from build123d import *

# Parameters (mm, degrees)
SKETCH_1_R               = 72.5
SKETCH_1_R_2             = 65
EXTRUDE_1_DEPTH          = 1
SKETCH_2_W               = 1
SKETCH_2_H               = 0.5
SKETCH_3_R               = 67.173254354
CUT_EXTRUDE_1_DEPTH      = 500
EXTRUDE_START            = 6
SKETCH_4_R               = 69.173254354
SKETCH_4_R_2             = 67.173254354
EXTRUDE_2_DEPTH          = 6
SKETCH_9_R               = 3
CUT_EXTRUDE_3_DEPTH      = 50
PATTERN_CIRCULAR_1_COUNT = 8
EXTRUDE_4_REACH          = 105.351
SKETCH_10_R              = 64.083899557
SKETCH_10_R_2            = 42.5
SKETCH_11_R              = 3
CUT_EXTRUDE_4_DEPTH      = 50
PATTERN_CIRCULAR_2_COUNT = 8
EXTRUDE_START_2          = -1
SKETCH_13_R              = 3
SKETCH_13_R_2            = 1.5
EXTRUDE_5_DEPTH          = 1
PATTERN_CIRCULAR_3_COUNT = 8
CUT_EXTRUDE_5_DEPTH      = 1
PATTERN_CIRCULAR_4_COUNT = 4


with BuildPart() as part:
    # 草图1 → 凸台-拉伸1 (new body)
    with BuildSketch(Plane(origin=(0, 0, 0), x_dir=(1, 0, 0), z_dir=(0, 1, 0))):
        with Locations(Location((0, 0, 0), (0, 0, 270))):
            Circle(SKETCH_1_R)
        with Locations(Location((0, 0, 0), (0, 0, 270))):
            Circle(SKETCH_1_R_2, mode=Mode.SUBTRACT)
    extrude(amount=EXTRUDE_1_DEPTH)

    # 草图2 → 旋转1 (revolve)
    with BuildSketch(Plane.XY, mode=Mode.PRIVATE) as revolve_1_sk:
        with Locations((-72, 1.25)):
            Rectangle(SKETCH_2_W, SKETCH_2_H)
    revolve(revolve_1_sk.sketch.rotate(Axis((0, 15.807831018, 0), (0, -1, 0)), 270), axis=Axis((0, 15.807831018, 0), (0, -1, 0)))

    # 草图3 → 切除-拉伸1 (cut)
    with BuildSketch(Plane(origin=(0, 1, 0), x_dir=(1, 0, 0), z_dir=(0, 1, 0))):
        with Locations(Location((0, 0, 0), (0, 0, 270))):
            Circle(SKETCH_3_R)
    extrude(amount=-CUT_EXTRUDE_1_DEPTH, mode=Mode.SUBTRACT)

    # 草图4 → 凸台-拉伸2 (add)
    with BuildSketch(Plane(origin=(0, 1, 0), x_dir=(1, 0, 0), z_dir=(0, 1, 0)).offset(EXTRUDE_START)):
        with Locations(Location((0, 0, 0), (0, 0, 270))):
            Circle(SKETCH_4_R)
        with Locations(Location((0, 0, 0), (0, 0, 270))):
            Circle(SKETCH_4_R_2, mode=Mode.SUBTRACT)
    extrude(amount=-EXTRUDE_2_DEPTH)

    # 草图5 → 旋转3 (revolve)
    with BuildSketch(Plane.XY, mode=Mode.PRIVATE) as revolve_3_sk:
        Polygon((-69.173254354, 7), (-62.5, 16.5), (-45.358003893, 16.5), (-42.5, 14.5), (-61.460773767, 14.5), (-66.729132467, 7), align=None)
    revolve(revolve_3_sk.sketch.rotate(Axis((0, 1.5, 0), (0, 1, 0)), 270), axis=Axis((0, 1.5, 0), (0, 1, 0)))

    # 草图9 → 切除-拉伸3 (cut)
    with BuildSketch(Plane(origin=(0, 16.5, 0), x_dir=(1, 0, 0), z_dir=(0, 1, 0))):
        with Locations(Location((25.043627949, 45.572104397, 0), (0, 0, 270))):
            Circle(SKETCH_9_R)
    cut_extrude_3 = extrude(amount=-CUT_EXTRUDE_3_DEPTH, mode=Mode.SUBTRACT)

    # 阵列(圆周)1: 切除-拉伸3 ×8 about axis
    pattern_circular_1_axis = Axis((0, 0, 0), (0, 1, 0))
    for i in range(1, PATTERN_CIRCULAR_1_COUNT):
        add(cut_extrude_3.rotate(pattern_circular_1_axis, i * 360 / PATTERN_CIRCULAR_1_COUNT), mode=Mode.SUBTRACT)

    # 凸台-拉伸4: up to this face of the body (flat: up to its plane)
    extrude_4_end = Plane(part.part.faces().sort_by_distance((0, 14.5, 59.72240057))[0])
    # 草图10 → 凸台-拉伸4 (add, up to the picked face)
    with BuildSketch(Plane.XZ.offset(-13), mode=Mode.PRIVATE) as extrude_4_sk1:
        with Locations(Location((0, 0, 0), (0, 0, 270))):
            Circle(SKETCH_10_R)
        with Locations(Location((0, 0, 0), (0, 0, 270))):
            Circle(SKETCH_10_R_2, mode=Mode.SUBTRACT)
    extrude_4_tool1 = split(extrude(extrude_4_sk1.sketch, amount=-EXTRUDE_4_REACH, mode=Mode.PRIVATE), bisect_by=extrude_4_end, keep=Keep.BOTH, mode=Mode.PRIVATE)
    add(extrude_4_tool1.solids().sort_by(Axis((0, 13, 62.271333), (0, 1, 0)))[0])

    # 草图11 → 切除-拉伸4 (cut)
    with BuildSketch(Plane(origin=(0, 16.5, 0), x_dir=(1, 0, 0), z_dir=(0, 1, 0))):
        with Locations(Location((14.515824903, -49.9328632, 0), (0, 0, 135))):
            Circle(SKETCH_11_R)
    cut_extrude_4 = extrude(amount=-CUT_EXTRUDE_4_DEPTH, mode=Mode.SUBTRACT)

    # 阵列(圆周)2: 切除-拉伸4 ×8 about axis
    pattern_circular_2_axis = Axis((0, 0, 0), (0, 1, 0))
    for i in range(1, PATTERN_CIRCULAR_2_COUNT):
        add(cut_extrude_4.rotate(pattern_circular_2_axis, i * 360 / PATTERN_CIRCULAR_2_COUNT), mode=Mode.SUBTRACT)

    # 草图12 → 切除-旋转1 (revolve, cut)
    with BuildSketch(Plane.XY, mode=Mode.PRIVATE) as cut_revolve_1_sk:
        Polygon((-69.173254354, 7), (-62.5, 16.5), (-70.752238468, 16.5), align=None)
    revolve(cut_revolve_1_sk.sketch.rotate(Axis((0, 0, 0), (0, 1, 0)), 270), axis=Axis((0, 0, 0), (0, 1, 0)), mode=Mode.SUBTRACT)

    # 草图13 → 凸台-拉伸5 (add)
    with BuildSketch(Plane.XZ.offset(-13).offset(EXTRUDE_START_2)):
        with Locations(Location((49.9328632, -14.515824903, 0), (0, 0, 135))):
            Circle(SKETCH_13_R)
        with Locations(Location((49.9328632, -14.515824903, 0), (0, 0, 270))):
            Circle(SKETCH_13_R_2, mode=Mode.SUBTRACT)
    extrude_5 = extrude(amount=EXTRUDE_5_DEPTH)

    # 阵列(圆周)3: 凸台-拉伸5 ×8 about axis
    pattern_circular_3_axis = Axis((0, 0, 0), (0, 1, 0))
    for i in range(1, PATTERN_CIRCULAR_3_COUNT):
        add(extrude_5.rotate(pattern_circular_3_axis, i * 360 / PATTERN_CIRCULAR_3_COUNT))

    # 草图14 → 切除-拉伸5 (cut)
    with BuildSketch(Plane(origin=(0, 16.5, 0), x_dir=(1, 0, 0), z_dir=(0, 1, 0))):
        with BuildLine():
            ThreePointArc((-15.741399661, 57.790873535), (-27.876499993, 53.013936615), (-38.69003161, 45.723715743))
            ThreePointArc((-38.69003161, 45.723715743), (-38.921101796, 42.950560173), (-36.147946226, 42.719489986))
            ThreePointArc((-36.147946226, 42.719489986), (-26.044905646, 49.530715026), (-14.707128549, 53.993788632))
            ThreePointArc((-14.707128549, 53.993788632), (-13.325721654, 56.40946664), (-15.741399661, 57.790873535))
        make_face()
    cut_extrude_5 = extrude(amount=-CUT_EXTRUDE_5_DEPTH, mode=Mode.SUBTRACT)

    # 阵列(圆周)4: 切除-拉伸5 ×4 about axis
    pattern_circular_4_axis = Axis((0, 0, 0), (0, 1, 0))
    for i in range(1, PATTERN_CIRCULAR_4_COUNT):
        add(cut_extrude_5.rotate(pattern_circular_4_axis, i * 360 / PATTERN_CIRCULAR_4_COUNT), mode=Mode.SUBTRACT)


solid = part.part
Build history of the part. All positions in model axes, mm. A direction names the side the tool comes from. Round coordinates to 2 decimals unless told otherwise and drop trailing zeros. Order: outer loops, then holes, each group sorted by start corner. A loop starts at its lowest first (then second) coordinate and runs counter-clockwise, first axis right, second up. Notation, with made-up numbers: M -6.5,-24.5 L 52.5,-24.5 A36 cw 52.5,13.5 Z; hole C 25,52 d11. An arc over 180 degrees is marked long. Use CSV: the item, a comma, the result in double quotes. Start each with the question number.
(1) Drill centre lines: probe 1 along Z at (x, y) = (38, 1.25); probe 2 along X at (y, z) = (14.75, 25); probe 3 along Y at (x, z) = (59, 3). Where is each one in solid material? Low to high.
(2) Cut at C-C on y = 3.5. List the corners of the cut face in (x, z).
(3) Cut at B-B on z = 0. List the corners of the cut face in (x, y), then the cut area to 3 significant figures.
(4) Cut at A-A on x = 0. List the corners of the cut face in (y, z), then the cut area to 3 significant figures.
(5) Flat gauge pins, fed straight in: P1, Ø5.5, axis at x = 25.04, z = -45.57, coming from the -Y side; P2, Ø3, axis at x = -34.5, y = 13, coming from the +Z side; P3, Ø6, axis at y = 5, z = -25.5, coming from the -X side; P4, Ø2.5, axis at x = -49.93, z = 14.52, coming from the +Y side. Where does each tip first touch, or does it go through?
(6) Mould opens along Z. For faces 1 (the face through (-47, 14, -26)), 2 (the face through (-42, 16.5, -18)) say: +Z half, -Z half, draft (parallel to the pull), parting line (faces both ways), or undercut.
(7) Tool access for faces 3 (the face through (42.8, 15.3, 23.9)), 4 (the face through (20.18, 3.55, 64.07)), 5 (the face through (-25.861, 13.74, 33.727)): list every direction of +Z, -Z, +X, -X, +Y, -Y with a clear straight run to the whole face (end or side of a thin tool).
Findings:
1,probe 1,"z = -61.74 to -60.57, -57.8 to -55.39, 55.39 to 57.8, 60.57 to 61.74"
1,probe 2,"x = -58.62 to -34.81, 34.81 to 42.57, 48.57 to 58.62"
1,probe 3,"y = 13 to 16.5"
2,outline,"C 0,0 d138.35; hole C 0,0 d134.35"
3,outline,"M -72.5,0 L -67.17,0 L -67.17,7 L -66.73,7 L -62.51,13 L -42.5,13 L -42.5,14.5 L -45.36,16.5 L -62.5,16.5 L -69.17,7 L -69.17,1 L -71.5,1 L -71.5,1.5 L -72.5,1.5 Z; M 42.5,13 L 62.51,13 L 66.73,7 L 67.17,7 L 67.17,0 L 72.5,0 L 72.5,1.5 L 71.5,1.5 L 71.5,1 L 69.17,1 L 69.17,7 L 62.5,16.5 L 45.36,16.5 L 42.5,14.5 Z"
3,area,"208 mm^2"
4,outline,"M 0,-72.5 L 1.5,-72.5 L 1.5,-71.5 L 1,-71.5 L 1,-69.17 L 7,-69.17 L 16.5,-62.5 L 16.5,-45.36 L 14.5,-42.5 L 13,-42.5 L 13,-62.51 L 7,-66.73 L 7,-67.17 L 0,-67.17 Z; M 0,67.17 L 7,67.17 L 7,66.73 L 13,62.51 L 13,42.5 L 14.5,42.5 L 16.5,45.36 L 16.5,62.5 L 7,69.17 L 1,69.17 L 1,71.5 L 1.5,71.5 L 1.5,72.5 L 0,72.5 Z"
4,area,"208 mm^2"
5,P1,"stops at y = 13"
5,P2,"stops at z = 56.58"
5,P3,"stops at x = -65.41"
5,P4,"passes through"
6,face 1,"undercut"
6,face 2,"draft"
7,face 3,"+Y"
7,face 4,"-Y"
7,face 5,"+Y, -Y"
